```python
from build123d import *

# Parameters (mm, degrees)
F0_R     = 14.2875
F0_R_2   = 3.175
F0_R_3   = 18.542
F1_DEPTH = 6.35
F2_R     = 6.35


with BuildPart() as f1:
    # F0 (on Right) → F1 (new body)
    with BuildSketch(Plane.YZ):
        Polygon((0, 406.4), (0, 0), (101.6, 0), (101.6, 152.4), (101.6, 190.5), (101.6, 406.4), align=None)
        with BuildLine():
            ThreePointArc((14.868026, 8.518026), (13.483992, 8.242724), (12.7, 9.416051))
            Line((12.7, 9.416051), (12.7, 36.83))
            ThreePointArc((12.7, 36.83), (13.071974, 37.728026), (13.97, 38.1))
            Line((13.97, 38.1), (41.383949, 38.1))
            ThreePointArc((41.383949, 38.1), (42.557276, 37.316008), (42.281974, 35.931974))
            Line((42.281974, 35.931974), (14.868026, 8.518026))
        make_face(mode=Mode.SUBTRACT)
        with BuildLine():
            Line((41.383949, 50.8), (13.97, 50.8))
            ThreePointArc((13.97, 50.8), (13.071974, 51.171974), (12.7, 52.07))
            Line((12.7, 52.07), (12.7, 79.483949))
            ThreePointArc((12.7, 79.483949), (13.483992, 80.657276), (14.868026, 80.381974))
            Line((14.868026, 80.381974), (42.281974, 52.968026))
            ThreePointArc((42.281974, 52.968026), (42.557276, 51.583992), (41.383949, 50.8))
        make_face(mode=Mode.SUBTRACT)
        with BuildLine():
            Line((88.9, 36.83), (88.9, 9.416051))
            ThreePointArc((88.9, 9.416051), (88.116008, 8.242724), (86.731974, 8.518026))
            Line((86.731974, 8.518026), (59.318026, 35.931974))
            ThreePointArc((59.318026, 35.931974), (59.042724, 37.316008), (60.216051, 38.1))
            Line((60.216051, 38.1), (87.63, 38.1))
            ThreePointArc((87.63, 38.1), (88.528026, 37.728026), (88.9, 36.83))
        make_face(mode=Mode.SUBTRACT)
        with BuildLine():
            ThreePointArc((60.216051, 50.8), (59.042724, 51.583992), (59.318026, 52.968026))
            Line((59.318026, 52.968026), (86.731974, 80.381974))
            ThreePointArc((86.731974, 80.381974), (88.116008, 80.657276), (88.9, 79.483949))
            Line((88.9, 79.483949), (88.9, 52.07))
            ThreePointArc((88.9, 52.07), (88.528026, 51.171974), (87.63, 50.8))
            Line((87.63, 50.8), (60.216051, 50.8))
        make_face(mode=Mode.SUBTRACT)
        with BuildLine():
            ThreePointArc((14.868026, 97.418026), (13.483992, 97.142724), (12.7, 98.316051))
            Line((12.7, 98.316051), (12.7, 125.73))
            ThreePointArc((12.7, 125.73), (13.071974, 126.628026), (13.97, 127))
            Line((13.97, 127), (41.383949, 127))
            ThreePointArc((41.383949, 127), (42.557276, 126.216008), (42.281974, 124.831974))
            Line((42.281974, 124.831974), (14.868026, 97.418026))
        make_face(mode=Mode.SUBTRACT)
        with BuildLine():
            Line((41.383949, 139.7), (13.97, 139.7))
            ThreePointArc((13.97, 139.7), (13.071974, 140.071974), (12.7, 140.97))
            Line((12.7, 140.97), (12.7, 168.383949))
            ThreePointArc((12.7, 168.383949), (13.483992, 169.557276), (14.868026, 169.281974))
            Line((14.868026, 169.281974), (42.281974, 141.868026))
            ThreePointArc((42.281974, 141.868026), (42.557276, 140.483992), (41.383949, 139.7))
        make_face(mode=Mode.SUBTRACT)
        with BuildLine():
            ThreePointArc((14.868026, 186.318026), (13.483992, 186.042724), (12.7, 187.216051))
            Line((12.7, 187.216051), (12.7, 214.63))
            ThreePointArc((12.7, 214.63), (13.071974, 215.528026), (13.97, 215.9))
            Line((13.97, 215.9), (41.383949, 215.9))
            ThreePointArc((41.383949, 215.9), (42.557276, 215.116008), (42.281974, 213.731974))
            Line((42.281974, 213.731974), (14.868026, 186.318026))
        make_face(mode=Mode.SUBTRACT)
        with BuildLine():
            Line((88.9, 125.73), (88.9, 98.316051))
            ThreePointArc((88.9, 98.316051), (88.116008, 97.142724), (86.731974, 97.418026))
            Line((86.731974, 97.418026), (59.318026, 124.831974))
            ThreePointArc((59.318026, 124.831974), (59.042724, 126.216008), (60.216051, 127))
            Line((60.216051, 127), (87.63, 127))
            ThreePointArc((87.63, 127), (88.528026, 126.628026), (88.9, 125.73))
        make_face(mode=Mode.SUBTRACT)
        with BuildLine():
            ThreePointArc((60.216051, 139.7), (59.042724, 140.483992), (59.318026, 141.868026))
            Line((59.318026, 141.868026), (86.731974, 169.281974))
            ThreePointArc((86.731974, 169.281974), (88.116008, 169.557276), (88.9, 168.383949))
            Line((88.9, 168.383949), (88.9, 140.97))
            ThreePointArc((88.9, 140.97), (88.528026, 140.071974), (87.63, 139.7))
            Line((87.63, 139.7), (60.216051, 139.7))
        make_face(mode=Mode.SUBTRACT)
        with BuildLine():
            Line((88.9, 214.63), (88.9, 187.216051))
            ThreePointArc((88.9, 187.216051), (88.116008, 186.042724), (86.731974, 186.318026))
            Line((86.731974, 186.318026), (59.318026, 213.731974))
            ThreePointArc((59.318026, 213.731974), (59.042724, 215.116008), (60.216051, 215.9))
            Line((60.216051, 215.9), (87.63, 215.9))
            ThreePointArc((87.63, 215.9), (88.528026, 215.528026), (88.9, 214.63))
        make_face(mode=Mode.SUBTRACT)
        with BuildLine():
            Line((41.383949, 228.6), (13.97, 228.6))
            ThreePointArc((13.97, 228.6), (13.071974, 228.971974), (12.7, 229.87))
            Line((12.7, 229.87), (12.7, 257.283949))
            ThreePointArc((12.7, 257.283949), (13.483992, 258.457276), (14.868026, 258.181974))
            Line((14.868026, 258.181974), (42.281974, 230.768026))
            ThreePointArc((42.281974, 230.768026), (42.557276, 229.383992), (41.383949, 228.6))
        make_face(mode=Mode.SUBTRACT)
        with BuildLine():
            ThreePointArc((14.868026, 275.218026), (13.483992, 274.942724), (12.7, 276.116051))
            Line((12.7, 276.116051), (12.7, 303.53))
            ThreePointArc((12.7, 303.53), (13.071974, 304.428026), (13.97, 304.8))
            Line((13.97, 304.8), (41.383949, 304.8))
            ThreePointArc((41.383949, 304.8), (42.557276, 304.016008), (42.281974, 302.631974))
            Line((42.281974, 302.631974), (14.868026, 275.218026))
        make_face(mode=Mode.SUBTRACT)
        with BuildLine():
            ThreePointArc((60.216051, 228.6), (59.042724, 229.383992), (59.318026, 230.768026))
            Line((59.318026, 230.768026), (86.731974, 258.181974))
            ThreePointArc((86.731974, 258.181974), (88.116008, 258.457276), (88.9, 257.283949))
            Line((88.9, 257.283949), (88.9, 229.87))
            ThreePointArc((88.9, 229.87), (88.528026, 228.971974), (87.63, 228.6))
            Line((87.63, 228.6), (60.216051, 228.6))
        make_face(mode=Mode.SUBTRACT)
        with BuildLine():
            Line((88.9, 303.53), (88.9, 276.116051))
            ThreePointArc((88.9, 276.116051), (88.116008, 274.942724), (86.731974, 275.218026))
            Line((86.731974, 275.218026), (59.318026, 302.631974))
            ThreePointArc((59.318026, 302.631974), (59.042724, 304.016008), (60.216051, 304.8))
            Line((60.216051, 304.8), (87.63, 304.8))
            ThreePointArc((87.63, 304.8), (88.528026, 304.428026), (88.9, 303.53))
        make_face(mode=Mode.SUBTRACT)
        with BuildLine():
            ThreePointArc((13.97, 317.5), (13.071974, 317.871974), (12.7, 318.77))
            Line((12.7, 318.77), (12.7, 346.183949))
            ThreePointArc((12.7, 346.183949), (13.483992, 347.357276), (14.868026, 347.081974))
            Line((14.868026, 347.081974), (42.281974, 319.668026))
            ThreePointArc((42.281974, 319.668026), (42.557276, 318.283992), (41.383949, 317.5))
            Line((41.383949, 317.5), (13.97, 317.5))
        make_face(mode=Mode.SUBTRACT)
        with BuildLine():
            Line((12.7, 365.016051), (12.7, 392.43))
            ThreePointArc((12.7, 392.43), (13.071974, 393.328026), (13.97, 393.7))
            Line((13.97, 393.7), (41.383949, 393.7))
            ThreePointArc((41.383949, 393.7), (42.557276, 392.916008), (42.281974, 391.531974))
            Line((42.281974, 391.531974), (14.868026, 364.118026))
            ThreePointArc((14.868026, 364.118026), (13.483992, 363.842724), (12.7, 365.016051))
        make_face(mode=Mode.SUBTRACT)
        with BuildLine():
            Line((87.63, 317.5), (60.216051, 317.5))
            ThreePointArc((60.216051, 317.5), (59.042724, 318.283992), (59.318026, 319.668026))
            Line((59.318026, 319.668026), (86.731974, 347.081974))
            ThreePointArc((86.731974, 347.081974), (88.116008, 347.357276), (88.9, 346.183949))
            Line((88.9, 346.183949), (88.9, 318.77))
            ThreePointArc((88.9, 318.77), (88.528026, 317.871974), (87.63, 317.5))
        make_face(mode=Mode.SUBTRACT)
        with BuildLine():
            Line((60.216051, 393.7), (87.63, 393.7))
            ThreePointArc((87.63, 393.7), (88.528026, 393.328026), (88.9, 392.43))
            Line((88.9, 392.43), (88.9, 365.016051))
            ThreePointArc((88.9, 365.016051), (88.116008, 363.842724), (86.731974, 364.118026))
            Line((86.731974, 364.118026), (59.318026, 391.531974))
            ThreePointArc((59.318026, 391.531974), (59.042724, 392.916008), (60.216051, 393.7))
        make_face(mode=Mode.SUBTRACT)
        Polygon((101.6, 152.4), (101.6, 0), (228.6, 0), (228.6, 152.4), (139.7, 152.4), align=None)
        with Locations((146.05, 50.8)):
            Circle(F0_R, mode=Mode.SUBTRACT)
        with Locations((215.9, 12.7)):
            Circle(F0_R_2, mode=Mode.SUBTRACT)
        with Locations((152.4, 139.7)):
            Circle(F0_R_2, mode=Mode.SUBTRACT)
        with Locations((184.15, 114.3)):
            Circle(F0_R_3, mode=Mode.SUBTRACT)
        with Locations((215.9, 139.7)):
            Circle(F0_R_2, mode=Mode.SUBTRACT)
        with BuildLine():
            Line((101.6, 190.5), (101.6, 152.4))
            Line((101.6, 152.4), (139.7, 152.4))
            ThreePointArc((139.7, 152.4), (112.759232, 163.559232), (101.6, 190.5))
        make_face()
    extrude(amount=F1_DEPTH)

    # F2
    f2_edges = [f1.edges().sort_by_distance(p)[0] for p in [
        (3.175, 228.6, 0),
        (3.175, 228.6, 152.4),
        (3.175, 0, 0),
        (3.175, 0, 406.4),
        (3.175, 101.6, 406.4),
    ]]
    fillet(f2_edges, radius=F2_R)


solid = f1.part
```
Source: CAD feature listing. Evaluate the final solid. Frame: model axes, mm. A direction names the side the tool comes from. Give positions to 0.01 mm unless a question says otherwise; leave off trailing zeros. Write each loop counter-clockwise with the first axis right and the second up, starting at its lowest first coordinate (ties: lowest second). Pieces come first, ordered by that corner, then holes.
1. Section query B-B (z = 248). Return the cut outline in (x, y), then the cut area to 3 significant figures.
2. Section query C-C (y = 183). Return the cut outline in (x, z), then the cut area to 3 significant figures.
3. Access query for faces 4 (the face through (3.13, 28.38, 333.57)), 5 (the face through (6.35, 62, 161)). Directions: +Z, -Z, +X, -X, +Y, -Y. A direction counts if a zero-diameter tool reaches every point of the face in a straight line with its end or side. Return the directions, or none.
4. Section query A-A (z = 114.3). Return the cut outline in (x, y), then the cut area to 3 significant figures.
5. First-contact query: pin 1 (5.5 mm diameter, centred on y = 152.4, z = 139.7, fed in from +X); pin 2 (1.9 mm diameter, centred on x = 4, z = 272, fed in from +Y); pin 3 (3 mm diameter, centred on x = 3.5, y = 160.5, fed in from +Z). Flat tips, straight axial feed; report the tip coordinate or a pass-through.
6. Section query D-D (x = 3.5). Count the separate pieces of the cut face and the enclosed holes in it, then the cut area to 3 significant figures.
7. Pull-direction query (Z, two-part tool) for faces 1 (the face through (0, 62, 161)), 2 (the face through (3.13, 113.06, 163.26)), 3 (the face through (3.13, 28.77, 200.22)); classes: +Z half, -Z half, draft (parallel to the pull), parting line (faces both ways), or undercut.
8. Material intervals for line 1 along Z through (x, y) = (4, 215.9) (3 decimals); line 2 along Y through (x, z) = (0.5, 229.5); line 3 along Y through (x, z) = (4.5, 79.5), sorted ascending.
Output values:
1. outline: (0, 0) - (6.35, 0) - (6.35, 12.7) - (0, 12.7) - close; (0, 25.05) - (6.35, 25.05) - (6.35, 76.55) - (0, 76.55) - close; (0, 88.9) - (6.35, 88.9) - (6.35, 101.6) - (0, 101.6) - close
1. area: 488 mm2
2. outline: (0, 0) - (6.35, 0) - (6.35, 95.79) - (0, 95.79) - close; (0, 132.81) - (6.35, 132.81) - (6.35, 152.4) - (0, 152.4) - close
2. area: 733 mm2
3. face 4: +X, -X
3. face 5: +Z, -Z, +X, +Y, -Y
4. outline: (0, 0) - (6.35, 0) - (6.35, 12.7) - (0, 12.7) - close; (0, 31.75) - (6.35, 31.75) - (6.35, 69.85) - (0, 69.85) - close; (0, 88.9) - (6.35, 88.9) - (6.35, 165.61) - (0, 165.61) - close; (0, 202.69) - (6.35, 202.69) - (6.35, 228.6) - (0, 228.6) - close
4. area: 974 mm2
5. pin 1: passes through
5. pin 2: stops at y = 101.6
5. pin 3: stops at z = 152.4
6. separate pieces: 1
6. enclosed holes: 23
6. area: 50,100 mm2
7. face 1: draft
7. face 2: +Z half
7. face 3: undercut
8. line 1: z = 0 to 9.525, 15.875 to 136.525, 142.875 to 152.4
8. line 2: y = 0 to 12.76, 42.6 to 59, 88.84 to 101.6
8. line 3: y = 0 to 12.7, 15.75 to 85.85, 88.9 to 228.6
